Can you work these out from the drawing? Everything is in mm from the part's minimum corner. Round coordinates to 2 decimals unless told otherwise and drop trailing zeros. Loops run counter-clockwise (first coordinate to the right, second up) from the corner with the lowest first, then second, coordinate; pieces in that order, holes last. Notation, with made-up numbers: (64, 77) -> (94, 77) arc R10 cw to (94, 90) -> close; hole circle Ø5 at (54.5, 48). An arc over 180 degrees is marked (long way). One line per item, written item: value.
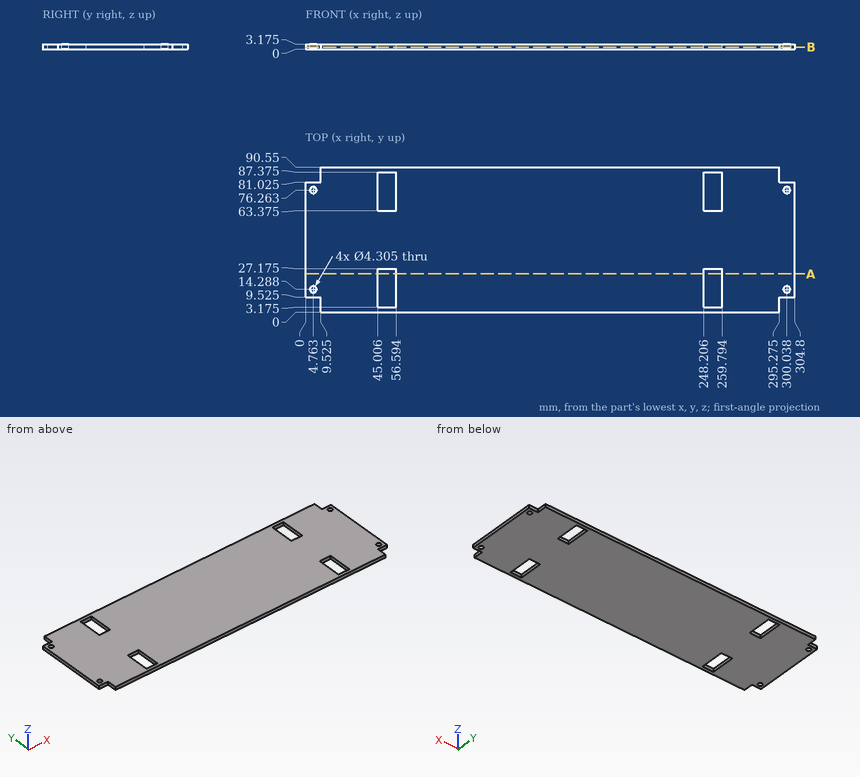
(1) Imagine slicing it at A-A on y = 24. Write out the boundary of the cut face in (x, z) (1 decimal).
Results below:
outline: (0, 0) -> (45, 0) -> (45, 3.2) -> (0, 3.2) -> close; (56.6, 0) -> (248.2, 0) -> (248.2, 3.2) -> (56.6, 3.2) -> close; (259.8, 0) -> (304.8, 0) -> (304.8, 3.2) -> (259.8, 3.2) -> close
(2) Imagine slicing it at B-B on z = 1.3. Give the number of separate pieces and of enclosed holes in the cut face, then the cut area to 3 significant figures.
Results below:
separate pieces: 1
enclosed holes: 8
area: 26,100 mm²
(3) For pin 1 Ø7 at (x, y) = (300.04, 76.26) entering from -Z; pin 2 Ø1.6 at (y, z) = (85, 1.5) entering from +X (1 decimal), each with a flat end and sliding along its axis, tell me the tip position at first contact or that it passes through.
Results below:
pin 1: stops at z = 0
pin 2: stops at x = 295.3
(4) Please list where these lines run through material, in increasing order: L1, parallel to X at y = 80, z = 1.7; L2, parallel to X at y = 85, z = 1.2 (1 decimal).
Results below:
L1: x = 0 to 45.01, 56.59 to 248.21, 259.79 to 304.8
L2: x = 9.5 to 45, 56.6 to 248.2, 259.8 to 295.3
